Geometry check sheet. Reference: the model listing, model coordinates, mm. Face numbers are marked on the shaded views. Give positions to 0.01 mm unless a question says otherwise; leave off trailing zeros. Loops run counter-clockwise (first coordinate to the right, second up) from the corner with the lowest first, then second, coordinate; pieces in that order, holes last.
1. Cross-section at D-D, the plane x = -8.75. Record the cut outline in (y, z).
2. Cross-section at C-C, the plane y = -32.5. Record the cut outline in (x, z) (1 decimal).
3. Cross-section at A-A, the plane z = 0. Record the cut outline in (x, y), plus the area to 3 significant figures.
4. Cross-section at B-B, the plane x = 0. Record the cut outline in (y, z).
5. Release check for a two-part mould opening along Z. For the marked faces 1 and 2 record: +Z half, -Z half, draft (parallel to the pull), parting line (faces both ways), or undercut.
6. Go/stop test with flat-tipped pins: pin 1 Ø1.5 at (y, z) = (26.5, -8) entering from +X; pin 2 Ø2 at (y, z) = (-6, -11.5) entering from +X; pin 3 Ø8 at (y, z) = (32, -8.5) entering from +X; pin 4 Ø4 at (y, z) = (-60.64, 0) entering from +X. Record where each tip stops, or that it passes through.
7. Material ranges on L1, parallel to Y at x = 12.3, z = 0; L2, parallel to X at y = 69, z = 0.5; L3, parallel to X at y = 7.5, z = -5.25, recorded low to high.
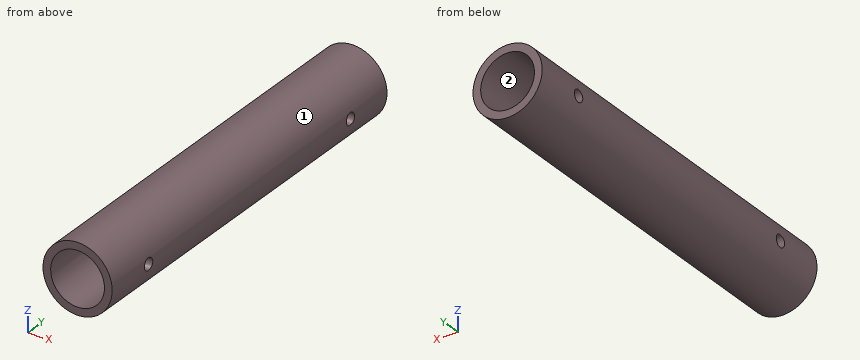
from build123d import *

# Parameters (mm, degrees)
SKETCH1_R           = 14.2875
SKETCH1_R_2         = 11.1125
BOSS_EXTRUDE1_DEPTH = 82.55
SKETCH2_R           = 2.4892
CUT_EXTRUDE1_DEPTH  = 85.986868471


with BuildPart() as part:
    # Sketch1 → Boss-Extrude1 (new, symmetric)
    with BuildSketch(Plane(origin=(0, 0, 0), x_dir=(1, 0, 0), z_dir=(0, 1, 0))):
        with Locations(Location((0, 0, 0), (0, 0, 270))):
            Circle(SKETCH1_R)
        with Locations(Location((0, 0, 0), (0, 0, 270))):
            Circle(SKETCH1_R_2, mode=Mode.SUBTRACT)
    extrude(amount=BOSS_EXTRUDE1_DEPTH, both=True)

    # Sketch2 → Cut-Extrude1 (cut, symmetric)
    with BuildSketch(Plane(origin=(0, 0, 0), x_dir=(0, 0, -1), z_dir=(1, 0, 0))):
        with Locations((0, 60.6425)):
            Circle(SKETCH2_R)
    cut_extrude1 = extrude(amount=CUT_EXTRUDE1_DEPTH, both=True, mode=Mode.SUBTRACT)

    # Mirror1: Cut-Extrude1 across plane
    add(cut_extrude1.mirror(Plane.ZX), mode=Mode.SUBTRACT)


solid = part.part
Result:
1. outline: (-82.55, -11.29) - (82.55, -11.29) - (82.55, -6.85) - (-82.55, -6.85) - close; (-82.55, 6.85) - (82.55, 6.85) - (82.55, 11.29) - (-82.55, 11.29) - close
2. outline: circle Ø28.6 at (0, 0); hole circle Ø22.2 at (0, 0)
3. outline: (-14.29, -82.55) - (-11.11, -82.55) - (-11.11, -63.13) - (-14.29, -63.13) - close; (-14.29, -58.15) - (-11.11, -58.15) - (-11.11, 58.15) - (-14.29, 58.15) - close; (-14.29, 63.13) - (-11.11, 63.13) - (-11.11, 82.55) - (-14.29, 82.55) - close; (11.11, -82.55) - (14.29, -82.55) - (14.29, -63.13) - (11.11, -63.13) - close; (11.11, -58.15) - (14.29, -58.15) - (14.29, 58.15) - (11.11, 58.15) - close; (11.11, 63.13) - (14.29, 63.13) - (14.29, 82.55) - (11.11, 82.55) - close
3. area: 985 mm2
4. outline: (-82.55, -14.29) - (82.55, -14.29) - (82.55, -11.11) - (-82.55, -11.11) - close; (-82.55, 11.11) - (82.55, 11.11) - (82.55, 14.29) - (-82.55, 14.29) - close
5. face 1: parting line
5. face 2: undercut
6. pin 1: stops at x = 12.31
6. pin 2: stops at x = 9.69
6. pin 3: stops at x = 13.56
6. pin 4: passes through
7. L1: y = -82.55 to -63.13, -58.15 to 58.15, 63.13 to 82.55
7. L2: x = -14.28 to -11.1, 11.1 to 14.28
7. L3: x = -13.29 to -9.79, 9.79 to 13.29
